The model under review builds one solid part; all positions refer to its coordinate system, in mm. A direction names the side the tool comes from. Round coordinates to 2 decimals unless told otherwise and drop trailing zeros. Loops run counter-clockwise (first coordinate to the right, second up) from the corner with the lowest first, then second, coordinate; pieces in that order, holes last. Notation, with made-up numbers: (36, 6.25) - (75, 6.25) arc R21 ccw to (75, 40.25) - close; hole circle Ø4 at (77.25, 43.25). An arc over 180 degrees is marked (long way). Answer as CSV lines item,"result".
from build123d import *

# Parameters (mm, degrees)
F0_W     = 90
F0_H     = 90
F1_DEPTH = 2.5
F2_W     = 90
F2_H     = 90
F2_R     = 41.5
F3_DEPTH = 2.5
F4_R     = 2.5
F5_DEPTH = 2.5


with BuildPart() as f1:
    # F0 (on Front) → F1 (new body)
    with BuildSketch(Plane.XZ):
        Rectangle(F0_W, F0_H)
    extrude(amount=F1_DEPTH)

    # F2 (on face) → F3 (join)
    with BuildSketch(Plane.XZ.offset(2.5)):
        Rectangle(F2_W, F2_H)
        Circle(F2_R, mode=Mode.SUBTRACT)
    extrude(amount=F3_DEPTH)

    # F4 (on face) → F5 (join)
    with BuildSketch(Plane.XZ.offset(2.5)):
        with Locations((0, 11.5)):
            Circle(F4_R)
    extrude(amount=F5_DEPTH)


solid = f1.part
1. Take a section at C-C (z = 0). State the section outline as (x, y) points, plus the area to 4 significant figures.
Numbers:
outline,"(-45, -5) - (-41.5, -5) - (-41.5, -2.5) - (41.5, -2.5) - (41.5, -5) - (45, -5) - (45, 0) - (-45, 0) - close"
area,"242.5 mm²"
2. Wall thickness on probe 1 along Z at (x, y) = (0, -4.3); probe 2 along Z at (x, y) = (0.5, -3.6); probe 3 along Y at (x, z) = (7, -20.5): over which ranges is each line inside the solid? List them lowest first.
Numbers:
probe 1,"z = -45 to -41.5, 9 to 14, 41.5 to 45"
probe 2,"z = -45 to -41.5, 9.05 to 13.95, 41.5 to 45"
probe 3,"y = -2.5 to 0"
3. Draft analysis for pull direction X (two halves, no side actions). For faces 3 (the face through (45, -2, -1)), 4 (the face through (-1, -2, 45)), 5 (the face through (39.584, -3.732, 12.465)), state which applies: +X half, -X half, draft (parallel to the pull), parting line (faces both ways), or undercut.
Numbers:
face 3,"+X half"
face 4,"draft"
face 5,"undercut"
4. Tool access review of faces 1 (the face through (-0.54, -3.73, 9.06)), 2 (the face through (-20.2, -5, -36.5)): name each direction out of +Z, -Z, +X, -X, +Y, -Y from which nothing blocks a thin tool from reaching the whole face with its end or side.
Numbers:
face 1,"-Y"
face 2,"+Z, -Z, +X, -X, -Y"
5. Take a section at A-A (y = -3.9). State the section outline as (x, z) points, plus the area to 3 significant figures.
Numbers:
outline,"(-45, -45) - (45, -45) - (45, 45) - (-45, 45) - close; circle Ø5 at (0, 11.5); hole circle Ø83 at (0, 0)"
area,"2,710 mm²"
6. Take a section at D-D (x = 23). State the section outline as (y, z) points, plus the area to 3 significant figures.
Numbers:
outline,"(-5, -45) - (0, -45) - (0, 45) - (-5, 45) - (-5, 34.54) - (-2.5, 34.54) - (-2.5, -34.54) - (-5, -34.54) - close"
area,"277 mm²"
7. Clearance check with a flat-ended pin moving along its axis: pin 1 (4 mm diameter, centred on x = 23, z = 24, fed in from -Y). State where the tip first meets the part, or that it passes through.
Numbers:
pin 1,"stops at y = -2.5"
8. Take a section at B-B (x = 0). State the section outline as (y, z) points, plus the area to 3 significant figures.
Numbers:
outline,"(-5, -45) - (0, -45) - (0, 45) - (-5, 45) - (-5, 41.5) - (-2.5, 41.5) - (-2.5, 14) - (-5, 14) - (-5, 9) - (-2.5, 9) - (-2.5, -41.5) - (-5, -41.5) - close"
area,"255 mm²"
